Here's how the part is built. I have some questions about the finished solid (model axes, mm). A direction names the side the tool comes from. Coordinates: 2 decimals unless noted, no trailing zeros. Write each loop counter-clockwise with the first axis right and the second up, starting at its lowest first coordinate (ties: lowest second). Pieces come first, ordered by that corner, then holes.
Item 1: We'd pull the mould along Y, two halves only. Please class faces 1 (the face through (-0.8, 0, -2.4)), 2 (the face through (0, 14, -6)), 3 (the face through (-2.1, 6, -2.5)): +Y half, -Y half, draft (parallel to the pull), parting line (faces both ways), or undercut.
Item 2: For faces 4 (the face through (-2.937, 25.285, -1.446)), 5 (the face through (-2.187, 2.958, -0.774)), 6 (the face through (-2.51, 14.49, -2.44)), 7 (the face through (-4, 27.75, -4)), 8 (the face through (-2.44, 1.48, -2.51)), which set-ups out of +Z, -Z, +X, -X, +Y, -Y let a thin tool reach every point of the face, with its end or its side?
Item 3: If I drill on line 1 (Y direction, x = -3.5, z = -4.25); line 2 (Y direction, x = -2.5, z = -2.75); line 3 (X direction, y = 1.25, z = -1.45), over which ranges is the centre line in solid material (lowest first)?
Item 4: If we section it at A-A (z = -4.25): Please give me the cut outline in (x, y), then the cut area to 3 significant figures.
Item 5: If we section it at B-B (y = 2.25): Please give me the cut outline in (x, z), then the cut area to 3 significant figures.
Item 6: If we section it at D-D (x = -6): Please give me the cut outline in (y, z).
Item 7: I'm going to push flat-ended pins straight in: pin 1 Ø2 at (x, z) = (-7, -4.5) entering from +Y; pin 2 Ø1.2 at (x, z) = (-2.5, -3) entering from +Y; pin 3 Ø4 at (y, z) = (10, -3.5) entering from -X. Where does each tip first touch, or does it pass through?
Item 8: If we section it at C-C (z = -2): Please give me the cut outline in (x, y).
Autodesk Inventor part; units mm, degrees
ref_plane "YZ Plane" through (0, 0, 0) normal (1, 0, 0) x (0, 1, 0)
ref_plane "XZ Plane" through (0, 0, 0) normal (0, 1, 0) x (-1, 0, 0)
ref_plane "XY Plane" through (0, 0, 0) normal (0, 0, 1) x (1, 0, 0)
sketch "Sketch1" plane through (0, 0, 0) normal (0, 1, 0) x (-1, 0, 0)
  line L0 (0, 0) -> (4.95, 0)
  line L1 (0, 0) -> (0, -4.95)
  line L2 (0, -4.95) -> (4.95, 0)
  dimension "d0" = 4.95
  dimension "d1" = 4.95
extrude "Extrusion1" add sketch "Sketch1" along normal blind 6
sketch "Sketch2" plane through (0, 6, 0) normal (0, 1, 0) x (1, 0, 0)
  line L0 (-4.95, 0) -> (0, 0)
  line L1 (0, 0) -> (-10, 0)
  line L2 (0, 0) -> (0, 10)
  line L3 (0, 10) -> (-10, 0)
  dimension "d4" = 10
  dimension "d5" = 10
extrude "Extrusion2" add sketch "Sketch2" along normal blind 2
sketch "Sketch3" plane through (0, 8, 0) normal (0, 1, 0) x (1, 0, 0)
  line L0 (-10, 0) -> (-4.95, 0)
  line L1 (-10, 0) -> (-4.95, 0)
  line L2 (0, 4.95) -> (0, 10)
  line L3 (-4.95, 0) -> (0, 4.95)
  line L4 (0, 4.95) -> (0, 10)
  line L5 (0, 10) -> (-10, 0)
  point P0 (0, 0)
extrude "Extrusion3" add sketch "Sketch3" along normal blind 19.75
sketch "Sketch4" plane through (0, 27.75, 0) normal (0, 1, 0) x (1, 0, 0)
  line L0 (-4.95, 0) -> (0, 0)
  line L1 (-4.95, 0) -> (0, 0)
  line L2 (-4.95, 0) -> (0, 4.95)
  line L3 (0, 0) -> (0, 4.95)
extrude "Extrusion4" add sketch "Sketch4" against normal blind 5
sketch "Sketch6" plane through (0, 27.75, 0) normal (0, 1, 0) x (1, 0, 0)
  line L0 (-10, 0) -> (-4.95, 0)
  line L1 (-10, 0) -> (0, 10)
  line L2 (0, 10) -> (-10, 0)
  line L3 (-4.95, 0) -> (0, 0)
  line L4 (0, 0) -> (0, 10)
  circle A0 centre (-2.6665, 2.6666) radius 1.25
  dimension "d12" = 2.5
  dimension "d17" = 3.3
  dimension "d18" = 2.6665
  dimension "d19" = 2.6666
extrude "Extrusion5" cut sketch "Sketch6" against normal blind 5 contours A0
sketch "Sketch7" plane through (0, 8, 0) normal (0, 1, 0) x (1, 0, 0)
  line L0 (0, 4.95) -> (-4.95, 0)
  line L1 (0, 4.95) -> (-4.95, 0)
  line L2 (0, 4.95) -> (-4.95, 0)
  line L3 (0, 0) -> (0, 4.95)
  line L4 (-4.95, 0) -> (0, 0)
  line L5 (0, 0) -> (0, 4.95)
extrude "Extrusion6" add sketch "Sketch7" along normal blind 2
sketch "Sketch8" plane through (0, 0, 0) normal (0, -1, 0) x (1, 0, 0)
  line L0 (-4.95, 0) -> (0, 0)
  line L1 (0, 0) -> (0, -4.95)
  circle A0 centre (-1.45, -1.45) radius 1
  dimension "d20" = 1.45
  dimension "d21" = 1.45
  dimension "d22" = 2
extrude "Extrusion7" cut sketch "Sketch8" against normal up to surface (10 mm away)
sketch "Sketch9" plane through (0, 27.75, 0) normal (0, 1, 0) x (1, 0, 0)
  line L0 (0, 10) -> (10.5977, -0.5977)
  line L1 (0, 0) -> (0, 10)
  line L2 (0, 10) -> (-10, 0)
  line L3 (0, 10) -> (11.6673, -1.6673)
  line L4 (11.6673, -1.6673) -> (1.6673, -11.6673)
  line L5 (11.6673, -1.6673) -> (30.5491, -1.6673) construction
  line L6 (-10, 0) -> (1.6673, -11.6673)
  arc A0 (8.435, -4.8995) -> (4.8995, -8.435) centre (6.6673, -6.6673) ccw
  line L7 (6.6673, -6.6673) -> (4.8995, -4.8995)
  circle A1 centre (4.8995, -4.8995) radius 1.25
  dimension "d25" = 45
  dimension "d26" = 16.5
  dimension "d27" = 135
  dimension "d28" = 5
  dimension "d29" = 2.5
sketch "Sketch10" plane through (0, 10, 0) normal (0, 1, 0) x (1, 0, 0)
  line L0 (-4.95, 0) -> (0, 0)
  line L1 (-4.95, 0) -> (0, 4.95)
  line L2 (0, 0) -> (0, 4.95)
  circle A0 centre (-1.45, 1.45) radius 1
  circle A1 centre (-1.45, 1.45) radius 1
  line L3 (0, 0) -> (0, 4.95)
  line L4 (-4.95, 0) -> (0, 4.95)
  line L5 (-4.95, 0) -> (0, 0)
extrude "Extrusion8" cut sketch "Sketch10" against normal blind 4
sketch "Sketch11" plane through (0, 6, 0) normal (0, -1, 0) x (1, 0, 0)
  line L0 (-3.3378, -1.6122) -> (-4.95, 0)
  line L1 (-1.6121, -3.3379) -> (-3.3378, -1.6122)
  line L2 (0, -4.95) -> (-1.6121, -3.3379)
  line L3 (0, -4.95) -> (0, 0)
  line L4 (0, 0) -> (0, -10)
  line L5 (0, -4.95) -> (0, -10)
  line L6 (-10, 0) -> (-4.95, 0)
  line L7 (-10, 0) -> (0, 0)
  line L8 (0, 0) -> (-4.95, 0)
  circle A0 centre (-1.45, -1.45) radius 1
  line L9 (0, -4.95) -> (0, 0)
  line L10 (0, 0) -> (-4.95, 0)
  line L11 (0, -4.95) -> (-4.95, 0)
  line L12 (0, -4.95) -> (-1.6121, -3.3379)
  line L13 (-1.6121, -3.3379) -> (-3.3378, -1.6122)
  line L14 (-3.3378, -1.6122) -> (-4.95, 0)
  line L15 (0, -4.95) -> (-4.95, 0)
  line L16 (0, -4.95) -> (0, -10)
  line L17 (0, 0) -> (0, -10)
  line L18 (0, -4.95) -> (0, 0)
  line L19 (0, 0) -> (-4.95, 0)
  line L20 (-10, 0) -> (0, 0)
  line L21 (-10, 0) -> (-4.95, 0)
  line L22 (0, -4.95) -> (-4.95, 0)
  line L23 (0, 0) -> (-4.95, 0)
  line L24 (0, -4.95) -> (0, 0)
  circle A1 centre (-1.45, -1.45) radius 1
  line L25 (0, -10) -> (-10, 0)
  line L26 (0, -10) -> (-10, 0)
  arc A2 (-1.6121, -3.3379) -> (-3.3378, -1.6122) centre (-2.6665, -2.6666) ccw
  arc A3 (-3.3378, -1.6122) -> (-1.6121, -3.3379) centre (-2.6665, -2.6666) ccw
  line L27 (-1.6121, -3.3379) -> (-3.3378, -1.6122)
  arc A4 (-3.3378, -1.6122) -> (-1.6121, -3.3379) centre (-2.6665, -2.6666) ccw
  circle A5 centre (-2.6665, -2.6666) radius 1.25
  arc A6 (-1.6121, -3.3379) -> (-3.3378, -1.6122) centre (-2.6665, -2.6666) ccw
  arc A7 (-3.3378, -1.6122) -> (-1.6121, -3.3379) centre (-2.6665, -2.6666) ccw
  circle A8 centre (-2.6665, -2.6666) radius 1.25
  line L28 (0, -10) -> (-10, 0)
  circle A9 centre (-2.6665, -2.6666) radius 1.25
  line L29 (0, 0) -> (0, -10)
  line L30 (0, -10) -> (-10, 0)
  line L31 (-10, 0) -> (0, 0)
  arc A10 (-1.6121, -3.3379) -> (-3.3378, -1.6122) centre (-2.6665, -2.6666) ccw
  line L32 (0, -4.95) -> (-1.6121, -3.3379)
  line L33 (0, -4.95) -> (0, 0)
  line L34 (0, 0) -> (-4.95, 0)
  line L35 (-3.3378, -1.6122) -> (-4.95, 0)
  line L36 (0, -4.95) -> (-4.95, 0)
  circle A11 centre (-1.45, -1.45) radius 1
  line L37 (0, 0) -> (0, -4.95)
  line L38 (-4.95, 0) -> (0, 0)
  line L39 (0, -4.95) -> (-4.95, 0)
  line L40 (0, -4.95) -> (-4.95, 0)
  circle A12 centre (-1.45, -1.45) radius 1
  circle A13 centre (-1.45, -1.45) radius 1
  line L41 (0, -4.95) -> (0, 0)
  line L42 (0, 0) -> (0, -4.95)
  line L43 (0, 0) -> (-4.95, 0)
  line L44 (-4.95, 0) -> (0, 0)
  circle A14 centre (-1.45, -1.45) radius 1
  line L45 (-4.95, 0) -> (0, 0)
  line L46 (0, -4.95) -> (-4.95, 0)
  line L47 (0, 0) -> (0, -4.95)
  line L48 (0, -4.95) -> (-4.95, 0)
  line L49 (-10, 0) -> (-4.95, 0)
  line L50 (0, -10) -> (-10, 0)
  line L51 (0, -4.95) -> (0, -10)
  line L52 (0, -10) -> (-10, 0)
  line L53 (0, 0) -> (0, -10)
  line L54 (0, -10) -> (-10, 0)
  line L55 (-3.3378, -1.6122) -> (-1.6121, -3.3379)
extrude "Extrusion9" add sketch "Sketch11" along normal blind 3 contours A3 L2 L4 L25 L6 L0 | L1 A3
properties part number "bracket servo_3DPrint"
Answer list:
1. face 1: -Y half
1. face 2: draft
1. face 3: undercut
2. face 4: +Y
2. face 5: -Y
2. face 6: +Z, +X
2. face 7: +Z, -Z, +X, -X, +Y
2. face 8: -Z, -X, -Y
3. line 1: y = 3 to 27.75
3. line 2: y = 3 to 22.75
3. line 3: x = -3.5 to -2.45, -0.45 to 0
4. outline: (-5.75, 3) - (-0.7, 3) - (-0.7, 0) - (0, 0) - (0, 6) - (-0.7, 6) - (-0.7, 22.75) - (0, 22.75) - (0, 27.75) - (-5.75, 27.75) - close
4. area: 133 mm2
5. outline: (-4.95, 0) - (0, -4.95) - (0, 0) - close; hole circle Ø2 at (-1.45, -1.45)
5. area: 9.11 mm2
6. outline: (3, -4) - (27.75, -4) - (27.75, 0) - (3, 0) - close
7. pin 1: passes through
7. pin 2: stops at y = 22.75
7. pin 3: stops at x = -8.5
8. outline: (-8, 3) - (-2.95, 3) - (-2.95, 0) - (-2.29, 0) - (-2.29, 6) - (-2.95, 6) - (-2.95, 22.75) - (-3.72, 22.75) - (-3.72, 27.75) - (-8, 27.75) - close; (-1.61, 22.75) - (0, 22.75) - (0, 27.75) - (-1.61, 27.75) - close; (-0.61, 0) - (0, 0) - (0, 6) - (-0.61, 6) - close
